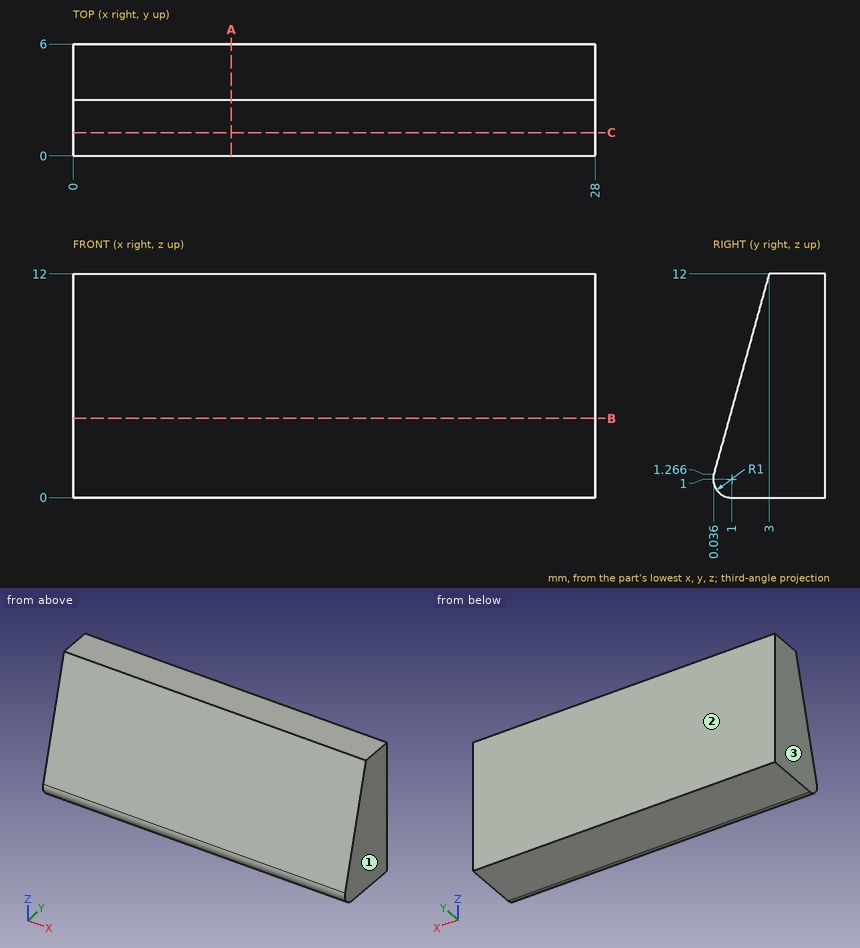
The figure shows three views and two pictorial views of one solid part (mm, origin at its lowest corner). Answer the questions. Round coordinates to 2 decimals unless told otherwise and drop trailing zeros. Order: outer loops, then holes, each group sorted by start corner. A loop starts at its lowest first (then second) coordinate and runs counter-clockwise, first axis right, second up. Notation, with made-up numbers: (62.5, 70.5) - (66.5, 70.5) arc R21 ccw to (66.5, 102.5) - close; hole circle Ø3 at (36.5, 25). An arc over 180 degrees is marked (long way). Write item = value, one per line. Start each with the question number.
1) Section B-B, the plane z = 4.25 is taken. Write down the section's boundary in (x, y).
2) Section C-C, the plane y = 1.25 is taken. Write down the section's boundary in (x, z), plus the area to 3 significant figures.
3) Section A-A, the plane x = 8.5 is taken. Write down the section's boundary in (y, z), plus the area to 3 significant figures.
4) For a pull along X with two mould halves and no side action, classify the marked faces 1, 2 and 3 as released by +X, released by -X, zero draft, split by the parting line, or undercut.
5) Straight lines are drawn through the part: L1, parallel to Y at x = 25.5, z = 1.25; L2, parallel to Y at x = 14.25, z = 4. For each, find the intervals that lie inside material, in ascending order.
6) Given pin 1 (1.5 mm diameter, centred on x = 16, z = 2, fed in from -Y), flat-ended and moving along its own axis, determine where the tip first touches the part or whether it passes through.
Results list:
q1.outline = (0, 0.86) - (28, 0.86) - (28, 6) - (0, 6) - close
q2.outline = (0, 0) - (28, 0) - (28, 5.66) - (0, 5.66) - close
q2.area = 159 mm^2
q3.outline = (0.04, 1.27) arc R1 ccw to (1, 0) - (6, 0) - (6, 12) - (3, 12) - close
q3.area = 55.5 mm^2
q4.face_1 = released by +X
q4.face_2 = zero draft
q4.face_3 = released by -X
q5.L1 = 0.03 to 6
q5.L2 = 0.79 to 6
q6.pin_1 = 0.03
